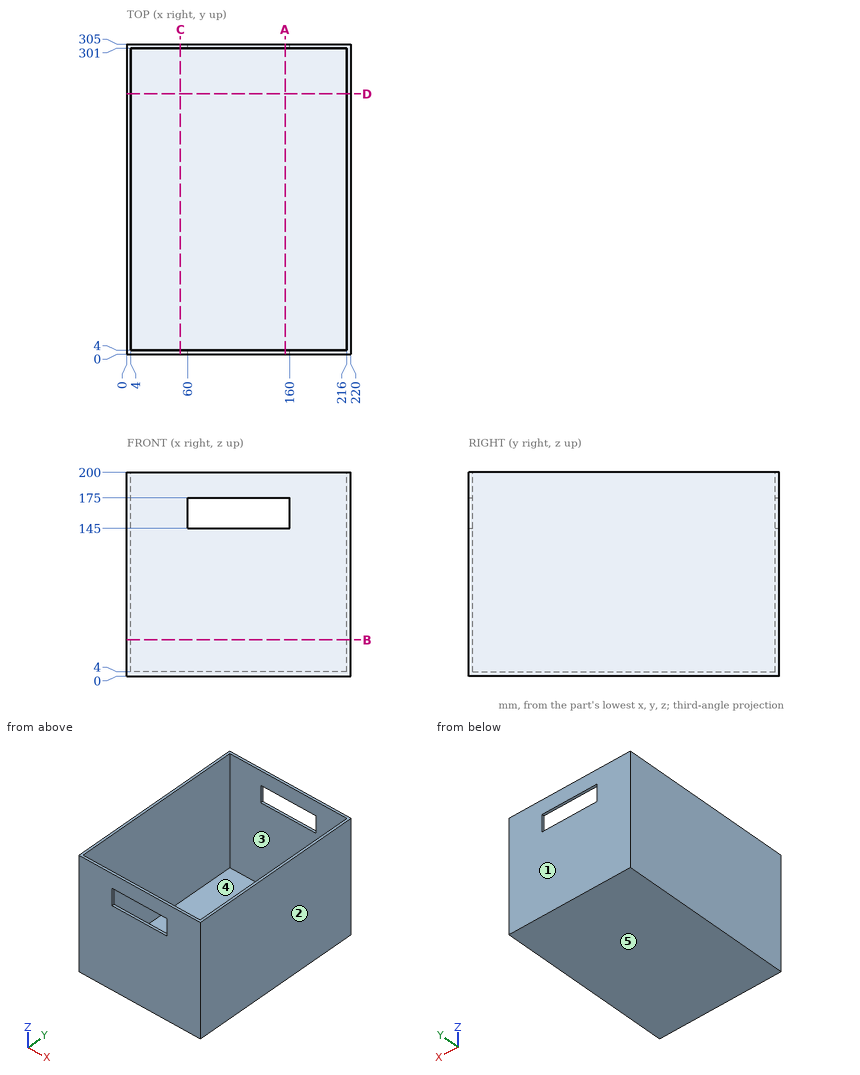
Input: dimensioned drawing with shaded views. Units: mm. Origin: part minimum x, y, z. A direction names the side the tool comes from. Coordinates: 2 decimals unless noted, no trailing zeros. Order: outer loops, then holes, each group sorted by start corner. A loop starts at its lowest first (then second) coordinate and runs counter-clockwise, first axis right, second up. Notation, with made-up numbers: (9.5, 73) - (41.5, 73) arc R19 ccw to (41.5, 106) - close; hole circle Ø1 at (2, 40.5). An arc over 180 degrees is marked (long way). One line per item, written item: value.
1) Cut plane A-A on x = 155.5. Output: boundary loops of the cut face in (y, z).
Computed values:
outline: (0, 0) - (305, 0) - (305, 145) - (301, 145) - (301, 4) - (4, 4) - (4, 145) - (0, 145) - close; (0, 175) - (4, 175) - (4, 200) - (0, 200) - close; (301, 175) - (305, 175) - (305, 200) - (301, 200) - close
2) Cut plane B-B on z = 35.5. Output: boundary loops of the cut face in (x, y).
Computed values:
outline: (0, 0) - (220, 0) - (220, 305) - (0, 305) - close; hole (4, 4) - (216, 4) - (216, 301) - (4, 301) - close
3) Cut plane D-D on y = 256. Output: boundary loops of the cut face in (x, z).
Computed values:
outline: (0, 0) - (220, 0) - (220, 200) - (216, 200) - (216, 4) - (4, 4) - (4, 200) - (0, 200) - close
4) Ray query, line 1 (Y direction, x = 39, z = 78); line 2 (X direction, y = 239, z = 143.5); line 3 (Z direction, x = 151, y = 261). Return the intervals inside material, ascending. Write a range as [from, to].
Computed values:
line 1: y = [0, 4], [301, 305]
line 2: x = [0, 4], [216, 220]
line 3: z = [0, 4]
5) Contact query for flat-ended pins moving along their axis: pin 1 (4.5 mm diameter, centred on x = 119.5, y = 2.5, fed in from -Z); pin 2 (12 mm diameter, centred on x = 180.5, y = 248, fed in from +Z). Output: stop coordinate, or through.
Computed values:
pin 1: stops at z = 0
pin 2: stops at z = 4
6) Reachability of the marked faces 4 and 5 from +Z, -Z, +X, -X, +Y, -Y: full face, straight path, thin tool, end or side. Return the list, or none.
Computed values:
face 4: +Z
face 5: -Z, +X, -X, +Y, -Y
7) Mould query, pull axis Y, two halves, no side actions, for the marked faces 1, 2 and 3. Classes: released by +Y, released by -Y, zero draft, split by the parting line, or undercut.
Computed values:
face 1: released by +Y
face 2: zero draft
face 3: undercut
8) Cut plane C-C on x = 52.5. Output: boundary loops of the cut face in (y, z).
Computed values:
outline: (0, 0) - (305, 0) - (305, 200) - (301, 200) - (301, 4) - (4, 4) - (4, 200) - (0, 200) - close
